Design review of the part built by this model. Coordinates are the model's own, in mm. Round coordinates to 2 decimals unless told otherwise and drop trailing zeros. Use a Markdown table: item, result.
Autodesk Inventor part; units mm, degrees
ref_plane "YZ Plane" through (0, 0, 0) normal (1, 0, 0) x (0, 1, 0)
ref_plane "XZ Plane" through (0, 0, 0) normal (0, 1, 0) x (-1, 0, 0)
ref_plane "XY Plane" through (0, 0, 0) normal (0, 0, 1) x (1, 0, 0)
sketch "Sketch1" plane through (0, 0, 0) normal (0, 1, 0) x (-1, 0, 0)
  line L0 (102.7304, -71.3481) -> (60.7304, -71.3481)
  line L1 (60.7304, -71.3481) -> (60.7304, 178.6519)
  line L2 (60.7304, 178.6519) -> (102.7304, 178.6519)
  line L3 (102.7304, 178.6519) -> (102.7304, -71.3481)
  point P0 (0, 0)
  dimension "d0" = 42
  dimension "d1" = 250
extrude "Plate1" add sketch "Sketch1" along normal blind 0.5
sketch "Sketch2" plane through (0, 0.5, 0) normal (0, 1, 0) x (1, 0, 0)
  line L0 (-102.7304, -178.6519) -> (-102.7304, 71.3481)
  line L1 (-60.7304, -178.6519) -> (-102.7304, -178.6519)
  point P0 (0, 0)
  point P1 (-81.7304, -148.6519)
  dimension "d3" = 21
  dimension "d4" = 30
hole "Hole1" at (-81.7304, 0.5, 148.6519) direction (0, -1, 0) diameter 6 depth 0.5 tip angle 118
equation "\"d10\" = Thickness"
equation "\"d2\" = Thickness"
equation "\"BendRadius\" = Thickness"
equation "\"BendReliefWidth\" = Thickness"
equation "\"BendReliefDepth\" = 0.5 * Thickness"
equation "\"CornerReliefSize\" = 4 * Thickness"
equation "\"MinimumRemnant\" = 2 * Thickness"
equation "\"TransitionRadius\" = BendRadius"
equation "\"JacobiRadiusSize\" = BendRadius"
equation "\"GapSize\" = Thickness"
properties part number "case"
1. Wall thickness on line 1 along Z through (x, y) = (-79, 0.25); line 2 along Z through (x, y) = (-82.5, 0.15): over which ranges is each line inside the solid? List them lowest first. Write a range as from..to.
Check values:
| item | result |
|---|---|
| line 1 | z = -71.35..147.41, 149.89..178.65 |
| line 2 | z = -71.35..145.75, 151.55..178.65 |
2. Insertion check: pin 1 (3.5 mm diameter, centred on x = -81.73, z = 148.65, fed in from +Y); pin 2 (4 mm diameter, centred on x = -90, z = -37.5, fed in from -Y). Each pin has a flat end and moves straight along its axis. Give the tip position at first contact, or say it passes through.
Check values:
| item | result |
|---|---|
| pin 1 | passes through |
| pin 2 | stops at y = 0 |
3. The part is to be moulded in two halves that separate along Z. For faces 1 (the face through (-82.632, 0.246, 151.513)), 2 (the face through (-81, 0.5, 55)), say which applies: pulls with the +Z half, pulls with the -Z half, needs draft (parallel to the pull), parting line crosses it, or undercut.
Check values:
| item | result |
|---|---|
| face 1 | undercut |
| face 2 | needs draft |
